Verification items for this drawing (mm, ordinates from the low corner). Round coordinates to 2 decimals unless told otherwise and drop trailing zeros. Order: outer loops, then holes, each group sorted by start corner. A loop starts at its lowest first (then second) coordinate and runs counter-clockwise, first axis right, second up. Notation, with made-up numbers: (31, 84) - (72, 84) arc R20 ccw to (72, 115) - close; hole circle Ø10 at (3.25, 89.25). An arc over 180 degrees is marked (long way). Answer as CSV lines item,"result". Start each with the question number.
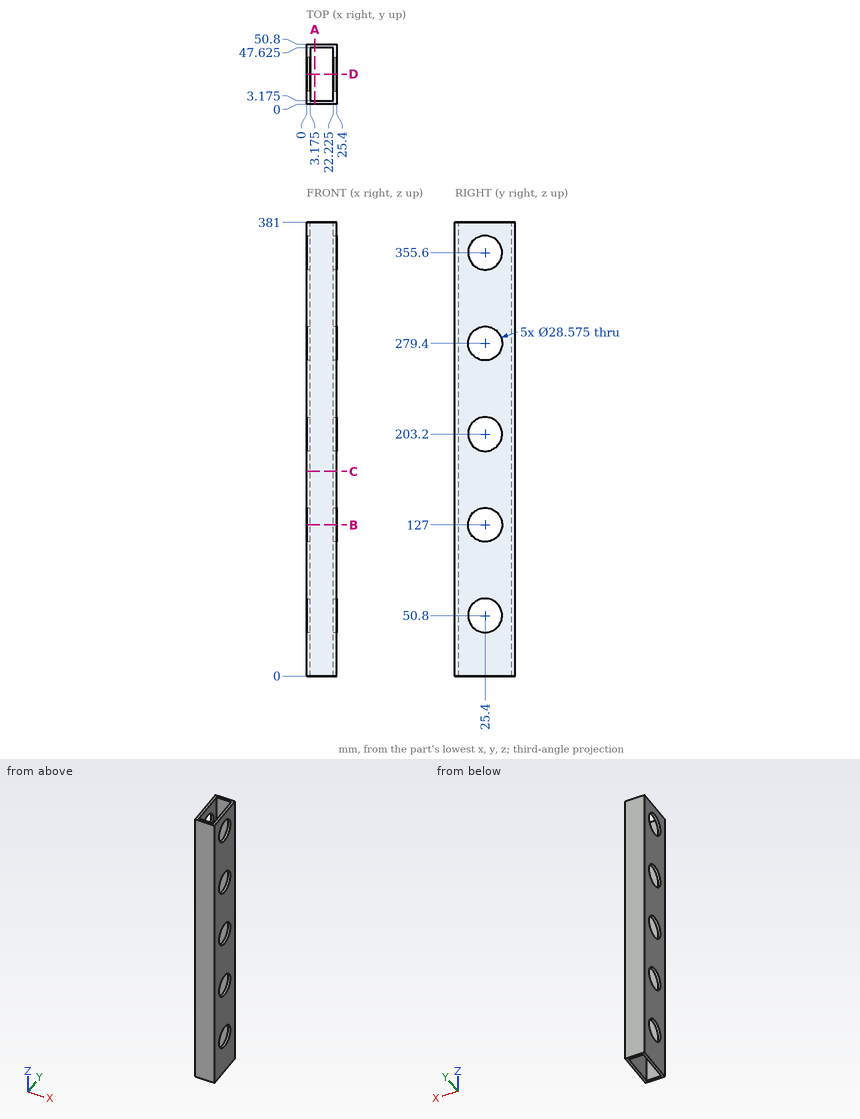
1. Go/stop test with flat-tipped pins: pin 1 Ø23 at (y, z) = (25.4, 279.4) entering from -X; pin 2 Ø13.5 at (y, z) = (23, 251.5) entering from -X. Record where each tip stops, or that it passes through.
2. Section check D-D on y = 25.4. Count the separate pieces of the cut face and the enclosed holes in it, plus the area to 3 significant figures.
3. Section check B-B on z = 127. Record the boundary of the cut face in (x, y) (1 decimal), plus the area to 3 significant figures.
4. Section check A-A on x = 7. Record the boundary of the cut face in (y, z) (3 decimals).
5. Thickness scan on probe 1 along X at (y, z) = (4.5, 281.5) (3 decimals); probe 2 along Y at (x, z) = (23.55, 127); probe 3 along Y at (x, z) = (21.25, 230) (3 decimals). Record the ranges inside material, lowest first.
6. Section check C-C on z = 172. Record the boundary of the cut face in (x, y) (3 decimals).
Numbers:
1,pin 1,"passes through"
1,pin 2,"stops at x = 0"
2,separate pieces,"12"
2,enclosed holes,"0"
2,area,"1,510 mm2"
3,outline,"(0, 0) - (25.4, 0) - (25.4, 11.1) - (22.2, 11.1) - (22.2, 3.2) - (3.2, 3.2) - (3.2, 11.1) - (0, 11.1) - close; (0, 39.7) - (3.2, 39.7) - (3.2, 47.6) - (22.2, 47.6) - (22.2, 39.7) - (25.4, 39.7) - (25.4, 50.8) - (0, 50.8) - close"
3,area,"262 mm2"
4,outline,"(0, 0) - (3.175, 0) - (3.175, 381) - (0, 381) - close; (47.625, 0) - (50.8, 0) - (50.8, 381) - (47.625, 381) - close"
5,probe 1,"x = 0 to 3.175, 22.225 to 25.4"
5,probe 2,"y = 0 to 11.11, 39.69 to 50.8"
5,probe 3,"y = 0 to 3.175, 47.625 to 50.8"
6,outline,"(0, 0) - (25.4, 0) - (25.4, 50.8) - (0, 50.8) - close; hole (3.175, 3.175) - (22.225, 3.175) - (22.225, 47.625) - (3.175, 47.625) - close"
